Could you check a few things on this model? Use its own coordinates, in mm. A direction names the side the tool comes from. Coordinates: 2 decimals unless noted, no trailing zeros. Loops run counter-clockwise (first coordinate to the right, second up) from the corner with the lowest first, then second, coordinate; pieces in that order, holes last. Notation, with made-up numbers: (5, -8.5) - (34, -8.5) arc R14 ccw to (34, 3.5) - close; hole circle Ø11 at (44, 81). An arc over 180 degrees is marked (long way). One line per item, written item: value. Start each with the question number.
(1) On a 3-axis mill with a long thin cutter (end or side, diameter ignored), from which of +Z, -Z, +X, -X, +Y, -Y can I reach the whole of each face in a straight line? I mean faces 4 (the face through (-14, -1, 5.53)), 5 (the face through (14.339, 40.496, -9.553)), 6 (the face through (-4.793, 38.424, -1.064)). Say none if no direction works.
(2) If we mould it in two halves opening along Z, with no side actions, what happens to faces 1 (the face through (-13.225, -1, 9)), 2 (the face through (0.45, 10.45, 1.43)), 3 (the face through (0, 24, 12.36))? For each: pulls with the +Z half, pulls with the -Z half, needs draft (parallel to the pull), parting line crosses it, or undercut.
(3) If we section it at A-A on z = 0: Write out the boundary of the cut face in (x, y) (3 decimals).
(4) If we section it at B-B on x = 0: Write out the boundary of the cut face in (y, z).
(5) If we section it at D-D on z = -9.5: Write out the boundary of the cut face in (x, y) (3 decimals), then the cut area to 3 significant figures.
(6) I'm going to push flat-ended pins straight in: P1, Ø12.5, axis at x = 1, z = -3.5, coming from the -Y side; P2, Ø2.5, axis at y = 6.87, z = 8.63, coming from the +X side (3 decimals); P3, Ø5, axis at x = 0, z = 0, coming from the +Y side. Where does each tip first touch, or does it pass through?
(7) If I drill on line 1 along Y through (x, z) = (14.2, -8.63); line 2 along Y through (x, z) = (-5, 3.5); line 3 along X through (y, z) = (22.8, 0) (3 decimals), over which ranges is the centre line in solid material (lowest first)? Write a range as from..to.
(8) If we section it at C-C on y = 42.27: Write out the boundary of the cut face in (x, z) (3 decimals).
```python
from build123d import *

# Parameters (mm, degrees)
BOSS_EXTRUDE1_DEPTH = 49.27
SKETCH12_W          = 2.099999999999998
SKETCH12_H          = 6.83
SKETCH12_W_2        = 2.0999999999999996
SKETCH12_H_2        = 6.829999999999998
SKETCH12_W_3        = 2.1000000000000014
BOSS_EXTRUDE2_DEPTH = 1.57
SKETCH4_R           = 4.91
CUT_EXTRUDE3_DEPTH  = 22
SKETCH5_R           = 2
CUT_EXTRUDE4_DEPTH  = 5
SKETCH7_R           = 1.5
CUT_EXTRUDE5_DEPTH  = 34.41594267711148
FILLET4_R           = 3
FILLET5_R           = 3
SKETCH13_R          = 2.000000000000001
SKETCH13_R_2        = 2
SKETCH13_R_3        = 2.0000000000000004
SKETCH13_R_4        = 1.9999999999999996
CUT_EXTRUDE6_DEPTH  = 2


with BuildPart() as part:
    # Sketch2 → Boss-Extrude1 (new body)
    with BuildSketch(Plane(origin=(0, 0, 0), x_dir=(1, 0, 0), z_dir=(0, 1, 0))):
        Polygon((-15.325000000000001, 12.36), (15.324999999999998, 12.36), (15.325, -12.360000000000003), (-15.324999999999996, -12.360000000000003), align=None)
    extrude(amount=BOSS_EXTRUDE1_DEPTH)

    # Sketch12 → Boss-Extrude2 (add)
    with BuildSketch(Plane.XZ):
        with Locations((-14.274999999999997, 8.945000000000004)):
            Rectangle(SKETCH12_W, SKETCH12_H)
        with Locations((-14.275000000000002, -8.944999999999999)):
            Rectangle(SKETCH12_W_2, SKETCH12_H_2)
        with Locations((14.274999999999999, 8.945000000000004)):
            Rectangle(SKETCH12_W_3, SKETCH12_H)
        with Locations((14.274999999999999, -8.944999999999999)):
            Rectangle(SKETCH12_W_3, SKETCH12_H_2)
    extrude(amount=BOSS_EXTRUDE2_DEPTH)

    # Sketch4 → Cut-Extrude3 (cut)
    with BuildSketch(Plane(origin=(0, 49.27, 0), x_dir=(1, 0, 0), z_dir=(0, 1, 0))):
        with Locations(Location((0, 0, 0), (0, 0, 270))):
            Circle(SKETCH4_R)
    extrude(amount=-CUT_EXTRUDE3_DEPTH, mode=Mode.SUBTRACT)

    # Sketch5 → Cut-Extrude4 (cut)
    with BuildSketch(Plane(origin=(0, 27.270000000000003, 0), x_dir=(1, 0, 0), z_dir=(0, 1, 0))):
        with Locations(Location((0, 0, 0), (0, 0, 270))):
            Circle(SKETCH5_R)
    extrude(amount=-CUT_EXTRUDE4_DEPTH, mode=Mode.SUBTRACT)

    # Sketch7 → Cut-Extrude5 (cut, through all)
    with BuildSketch(Plane(origin=(0, 22.270000000000003, 0), x_dir=(1, 0, 0), z_dir=(0, 1, 0))):
        with Locations(Location((0, 0, 0), (0, 0, 270))):
            Circle(SKETCH7_R)
    extrude(amount=-CUT_EXTRUDE5_DEPTH, mode=Mode.SUBTRACT)

    # Fillet4
    # the kernel refuses this fillet: 3 mm, written as the material it takes off along each edge
    with BuildSketch(Plane(origin=(0, 27.270000000000003, 0), x_dir=(-1.8e-16, 0, 1), z_dir=(-1, 0, -1.8e-16))) as fillet4_piece_1:
        with BuildLine():
            CenterArc((5, -2.9986496961132367), FILLET4_R, 91.7191313208778, 88.2808686791222)
            Line((2, -2.9986496961132367), (1.94, -2.9986496961132367))
            Line((1.94, -2.9986496961132367), (1.94, 0))
            Line((1.94, 0), (2, 0.05999999999999872))
            ThreePointArc((2, 0.05999999999999872), (3.455, 0.05999999999999872), (4.9082, 0.05997299392226552))
            Line((4.9082, 0.05997299392226552), (4.91, 0))
        make_face()
    revolve(axis=Axis((0, 27.270000000000003, 0), (0, 1, 0)), mode=Mode.SUBTRACT)

    # Fillet5
    # the kernel refuses this fillet: 3 mm, written as the material it takes off along each edge
    with BuildSketch(Plane(origin=(0, 22.270000000000003, 0), x_dir=(-1.8e-16, 0, 1), z_dir=(-1, 0, -1.8e-16))) as fillet5_piece_1:
        with BuildLine():
            CenterArc((4.5, -1.6583123951831418), FILLET5_R, 146.44269023799268, 33.55730976200732)
            Line((2.0000000000025064, -1.66267e-12), (1.9500000000025566, 0.03316624790196698))
            ThreePointArc((1.9500000000025566, 0.03316624790196698), (1.7500000000012532, 0.05999999999999872), (1.5, 0.05999999999999872))
            Line((1.5, 0.05999999999999872), (1.44, 0))
            Line((1.44, 0), (1.44, -1.6583123951831418))
            Line((1.44, -1.6583123951831418), (1.5, -1.6583123951831418))
        make_face()
    revolve(axis=Axis((0, 22.270000000000003, 0), (0, 1, 0)), mode=Mode.SUBTRACT)

    # Sketch13 → Cut-Extrude6 (cut)
    with BuildSketch(Plane(origin=(15.324999999999998, 0, -1.08e-15), x_dir=(-7e-17, 0, -1), z_dir=(1, 0, -7e-17))):
        with Locations((-8.630000000000006, 42.27)):
            Circle(SKETCH13_R)
        with Locations((8.629999999999999, 42.27)):
            Circle(SKETCH13_R_2)
        with Locations((-8.630000000000006, 6.870000000000001)):
            Circle(SKETCH13_R_3)
        with Locations((8.629999999999999, 6.870000000000001)):
            Circle(SKETCH13_R_4)
    extrude(amount=-CUT_EXTRUDE6_DEPTH, mode=Mode.SUBTRACT)


solid = part.part
```
Values:
1. face 4: +X, -X, -Y
1. face 5: +X
1. face 6: +Y
2. face 1: needs draft
2. face 2: undercut
2. face 3: pulls with the +Z half
3. outline: (-15.325, 0) - (-1.5, 0) - (-1.5, 20.612) arc R3 ccw to (-2, 22.27) - (-2, 24.271) arc R3 ccw to (-4.91, 27.27) - (-4.91, 49.27) - (-15.325, 49.27) - close; (1.5, 0) - (15.325, 0) - (15.325, 49.27) - (4.91, 49.27) - (4.91, 27.27) arc R3 ccw to (2, 24.271) - (2, 22.27) arc R3 ccw to (1.5, 20.612) - close
4. outline: (0, -12.36) - (49.27, -12.36) - (49.27, -4.91) - (27.27, -4.91) arc R3 ccw to (24.27, -2) - (22.27, -2) arc R3 ccw to (20.61, -1.5) - (0, -1.5) - close; (0, 1.5) - (20.61, 1.5) arc R3 ccw to (22.27, 2) - (24.27, 2) arc R3 ccw to (27.27, 4.91) - (49.27, 4.91) - (49.27, 12.36) - (0, 12.36) - close
5. outline: (-15.325, -1.57) - (-13.225, -1.57) - (-13.225, 0) - (13.225, 0) - (13.225, -1.57) - (15.325, -1.57) - (15.325, 5.069) - (13.325, 5.069) - (13.325, 8.671) - (15.325, 8.671) - (15.325, 40.469) - (13.325, 40.469) - (13.325, 44.071) - (15.325, 44.071) - (15.325, 49.27) - (-15.325, 49.27) - close
5. area: 1,500 mm2
6. P1: stops at y = 0
6. P2: stops at x = 13.325
6. P3: stops at y = 25.93
7. line 1: y = -1.57..4.87, 8.87..40.27, 44.27..49.27
7. line 2: y = 0..49.27
7. line 3: x = -15.325..-2, 2..15.325
8. outline: (-15.325, -12.36) - (15.325, -12.36) - (15.325, -10.63) - (13.325, -10.63) - (13.325, -6.63) - (15.325, -6.63) - (15.325, 6.63) - (13.325, 6.63) - (13.325, 10.63) - (15.325, 10.63) - (15.325, 12.36) - (-15.325, 12.36) - close; hole circle Ø9.82 at (0, 0)
